Build history of the part. All positions in model axes, mm. A direction names the side the tool comes from. Coordinates: 2 decimals unless noted, no trailing zeros. Order: outer loops, then holes, each group sorted by start corner. A loop starts at its lowest first (then second) coordinate and runs counter-clockwise, first axis right, second up. Notation, with made-up numbers: (48, 59) - (75, 59) arc R22 ccw to (75, 80) - close; hole circle Ø5 at (63, 28). An arc over 180 degrees is marked (long way). One line per item, written item: value.
from build123d import *

# Parameters (mm, degrees)
SKETCH_1_W                    = 30
SKETCH_1_H                    = 46
EXTRUDE_1_DEPTH               = 12.25
SKETCH_2_W                    = 9
SKETCH_2_H                    = 9.25
CUT_EXTRUDE_1_DEPTH           = 47
SKETCH_3_W                    = 9
SKETCH_3_H                    = 9.25
CUT_EXTRUDE_2_DEPTH           = 47
HOLE_WIZARD_M3_5_1_AT_2_COUNT = 2
HOLE_WIZARD_M3_5_1_AT_2_PITCH = 28


with BuildPart() as part:
    # 草图1 → 凸台-拉伸1 (new body)
    with BuildSketch(Plane.XZ.offset(6)):
        Rectangle(SKETCH_1_W, SKETCH_1_H)
    extrude(amount=-EXTRUDE_1_DEPTH)

    # 草图2 → 切除-拉伸1 (cut, through all)
    with BuildSketch(Plane(origin=(0, 0, -23), x_dir=(-1, 0, 0), z_dir=(0, 0, -1))):
        with Locations((10.5, -1.375)):
            Rectangle(SKETCH_2_W, SKETCH_2_H)
    extrude(amount=-CUT_EXTRUDE_1_DEPTH, mode=Mode.SUBTRACT)

    # 草图3 → 切除-拉伸2 (cut, through all)
    with BuildSketch(Plane(origin=(0, 0, -23), x_dir=(-1, 0, 0), z_dir=(0, 0, -1))):
        with Locations((-10.5, -1.375)):
            Rectangle(SKETCH_3_W, SKETCH_3_H)
    extrude(amount=-CUT_EXTRUDE_2_DEPTH, mode=Mode.SUBTRACT)

    # 草图4 → 旋转1 (revolve)
    with BuildSketch(Plane.XY.offset(19)):
        Polygon((6, -0.625), (6, -3.125), (10.5, -3.125), (10.5, -0.875), (9.5, -0.875), (9.5, -1.625), (7, -1.625), (7, -0.625), align=None)
    revolve(axis=Axis((6, -3.125, 19), (1, 0, 0)))

    # 草图5 → 旋转2 (revolve)
    with BuildSketch(Plane.XY.offset(19)):
        Polygon((-10.5, -0.875), (-10.5, -3.125), (-6, -3.125), (-6, -0.625), (-7, -0.625), (-7, -1.625), (-9.5, -1.625), (-9.5, -0.875), align=None)
    revolve(axis=Axis((-10.5, -3.125, 19), (1, 0, 0)))

    # 草图6 → 旋转3 (revolve)
    with BuildSketch(Plane.XY.offset(-19)):
        Polygon((6, -0.625), (6, -3.125), (10.5, -3.125), (10.5, -0.875), (9.5, -0.875), (9.5, -1.625), (7, -1.625), (7, -0.625), align=None)
    revolve(axis=Axis((6, -3.125, -19), (1, 0, 0)))

    # 草图7 → 旋转4 (revolve)
    with BuildSketch(Plane.XY.offset(-19)):
        Polygon((-10.5, -0.875), (-10.5, -3.125), (-6, -3.125), (-6, -0.625), (-7, -0.625), (-7, -1.625), (-9.5, -1.625), (-9.5, -0.875), align=None)
    revolve(axis=Axis((-10.5, -3.125, -19), (1, 0, 0)))

    # 草图8 → M3.5 平头机械螺钉的锥形沉头孔1 (revolve, cut)
    with BuildSketch(Plane(origin=(0, -6, -14), x_dir=(0, 0, -1), z_dir=(1, 0, 0))):
        Polygon((0, 0), (0, 12.25), (2.5, 12.25), (2.067, 11.817), (2.067, 0.433), (2.5, 0), align=None)
    hole_wizard_m3_5_1 = revolve(axis=Axis((0, -12.35, -14), (0, 1, 0)), mode=Mode.SUBTRACT)

    # M3.5 平头机械螺钉的锥形沉头孔1 at 2: M3.5 平头机械螺钉的锥形沉头孔1 ×2
    with Locations(*[(0, 0, i * HOLE_WIZARD_M3_5_1_AT_2_PITCH) for i in range(1, HOLE_WIZARD_M3_5_1_AT_2_COUNT)]):
        add(hole_wizard_m3_5_1, mode=Mode.SUBTRACT)


solid = part.part
1. Band-saw the part on D-D, the plane z = -2.5. Give the cut face in (x, y).
Values found:
outline: (-15, 3.25) - (-6, 3.25) - (-6, -6) - (6, -6) - (6, 3.25) - (15, 3.25) - (15, 6.25) - (-15, 6.25) - close
2. Band-saw the part on B-B, the plane z = 14. Give the cut face in (x, y).
Values found:
outline: (-15, 3.25) - (-6, 3.25) - (-6, -6) - (-2.5, -6) - (-2.07, -5.57) - (-2.07, 5.82) - (-2.5, 6.25) - (-15, 6.25) - close; (2.07, -5.57) - (2.5, -6) - (6, -6) - (6, 3.25) - (15, 3.25) - (15, 6.25) - (2.5, 6.25) - (2.07, 5.82) - close
3. Probe line 1 along Z through (x, y) = (0, 3.5); line 2 along X through (y, z) = (1.5, 14); line 3 along Y through (x, z) = (-7, 9). List the from-to ranges inside material, lowest first.
Values found:
line 1: z = -23 to -16.07, -11.93 to 11.93, 16.07 to 23
line 2: x = -6 to -2.07, 2.07 to 6
line 3: y = 3.25 to 6.25
4. Flat gauge pins, fed straight in: P1, Ø2, axis at y = -2, z = 18, coming from the +X side; P2, Ø4, axis at y = -3.5, z = -18.5, coming from the -X side; P3, Ø3, axis at y = -1.5, z = -4.5, coming from the -X side. Where does each tip first touch, or does it go through?
Values found:
P1: stops at x = 10.5
P2: stops at x = -10.5
P3: stops at x = -6
5. 3-axis set-ups, long thin cutter, end or side, ignore diameter. For faces 1 (the face through (-10, -3.6, 16.8)), 2 (the face through (8.232, -3.32, -17.513)), 3 (the face through (15, 5, 0)): which of +Z, -Z, +X, -X, +Y, -Y reach the whole face in a straight line?
Values found:
face 1: -X
face 2: none
face 3: +Z, -Z, +X, +Y, -Y
6. Band-saw the part on C-C, the plane y = 4.25. Give the cut face in (x, z).
Values found:
outline: (-15, -23) - (15, -23) - (15, 23) - (-15, 23) - close; hole circle Ø4.13 at (0, -14); hole circle Ø4.13 at (0, 14)
7. Band-saw the part on A-A, the plane x = 0. Give the cut face in (y, z), and give its area (3 significant figures).
Values found:
outline: (-6, -23) - (6.25, -23) - (6.25, -16.5) - (5.82, -16.07) - (-5.57, -16.07) - (-6, -16.5) - close; (-6, -11.5) - (-5.57, -11.93) - (5.82, -11.93) - (6.25, -11.5) - (6.25, 11.5) - (5.82, 11.93) - (-5.57, 11.93) - (-6, 11.5) - close; (-6, 16.5) - (-5.57, 16.07) - (5.82, 16.07) - (6.25, 16.5) - (6.25, 23) - (-6, 23) - close
area: 461 mm2
8. Two-plate mould, pull along Y, no slides. Class faces 4 (the face through (10, -3.6, -21.2)), 5 (the face through (-15, 5, 0)), 6 (the face through (0, -6, 0)): pulls with the +Y half, pulls with the -Y half, needs draft (parallel to the pull), parting line crosses it, or undercut.
Values found:
face 4: undercut
face 5: needs draft
face 6: pulls with the -Y half
